```python
from build123d import *

# Parameters (mm, degrees)
EXTRUDE_1_DEPTH     = 115
CUT_EXTRUDE_1_DEPTH = 118.951465627


with BuildPart() as part:
    # 草图1 → 凸台-拉伸1 (new body)
    with BuildSketch(Plane(origin=(0, 0, 0), x_dir=(1, 0, 0), z_dir=(0, 1, 0))):
        with BuildLine():
            Line((-1.042752475, -10.085861632), (3.857247525, -10.085861632))
            ThreePointArc((3.857247525, -10.085861632), (4.757247525, -10.985861632), (3.857247525, -11.885861632))
            Line((3.857247525, -11.885861632), (1.076161722, -11.885861632))
            ThreePointArc((1.076161722, -11.885861632), (0.722608332, -12.032308241), (0.576161722, -12.385861632))
            Line((0.576161722, -12.385861632), (0.576161722, -12.790788968))
            ThreePointArc((0.576161722, -12.790788968), (0.614221956, -12.982130685), (0.722608332, -13.144342359))
            Line((0.722608332, -13.144342359), (2.885447948, -15.307181975))
            ThreePointArc((2.885447948, -15.307181975), (3.858717994, -15.957500229), (5.006768291, -16.185861632))
            Line((5.006768291, -16.185861632), (8.907726758, -16.185861632))
            ThreePointArc((8.907726758, -16.185861632), (10.055777055, -15.957500229), (11.029047102, -15.307181975))
            Line((11.029047102, -15.307181975), (13.191886718, -13.144342359))
            ThreePointArc((13.191886718, -13.144342359), (13.300273094, -12.982130685), (13.338333327, -12.790788968))
            Line((13.338333327, -12.790788968), (13.338333327, -12.385861632))
            ThreePointArc((13.338333327, -12.385861632), (13.191886718, -12.032308241), (12.838333327, -11.885861632))
            Line((12.838333327, -11.885861632), (10.057247525, -11.885861632))
            ThreePointArc((10.057247525, -11.885861632), (9.157247525, -10.985861632), (10.057247525, -10.085861632))
            Line((10.057247525, -10.085861632), (14.957247525, -10.085861632))
            ThreePointArc((14.957247525, -10.085861632), (16.371461087, -10.671648069), (16.957247525, -12.085861632))
            Line((16.957247525, -12.085861632), (16.957247525, -16.985861632))
            ThreePointArc((16.957247525, -16.985861632), (16.057247525, -17.885861632), (15.157247525, -16.985861632))
            Line((15.157247525, -16.985861632), (15.157247525, -14.204775829))
            ThreePointArc((15.157247525, -14.204775829), (15.010800915, -13.851222438), (14.657247525, -13.704775829))
            Line((14.657247525, -13.704775829), (14.252320188, -13.704775829))
            ThreePointArc((14.252320188, -13.704775829), (14.060978472, -13.742836063), (13.898766797, -13.851222438))
            Line((13.898766797, -13.851222438), (11.735927181, -16.014062054))
            ThreePointArc((11.735927181, -16.014062054), (11.085608927, -16.987332101), (10.857247525, -18.135382398))
            Line((10.857247525, -18.135382398), (10.857247525, -22.036340865))
            ThreePointArc((10.857247525, -22.036340865), (11.085608927, -23.184391162), (11.735927181, -24.157661209))
            Line((11.735927181, -24.157661209), (13.898766797, -26.320500825))
            ThreePointArc((13.898766797, -26.320500825), (14.060978472, -26.4288872), (14.252320188, -26.466947434))
            Line((14.252320188, -26.466947434), (14.657247525, -26.466947434))
            ThreePointArc((14.657247525, -26.466947434), (15.010800915, -26.320500825), (15.157247525, -25.966947434))
            Line((15.157247525, -25.966947434), (15.157247525, -23.185861632))
            ThreePointArc((15.157247525, -23.185861632), (16.057247525, -22.285861632), (16.957247525, -23.185861632))
            Line((16.957247525, -23.185861632), (16.957247525, -28.085861632))
            ThreePointArc((16.957247525, -28.085861632), (16.371461087, -29.500075194), (14.957247525, -30.085861632))
            Line((14.957247525, -30.085861632), (10.057247525, -30.085861632))
            ThreePointArc((10.057247525, -30.085861632), (9.157247525, -29.185861632), (10.057247525, -28.285861632))
            Line((10.057247525, -28.285861632), (12.838333327, -28.285861632))
            ThreePointArc((12.838333327, -28.285861632), (13.191886718, -28.139415022), (13.338333327, -27.785861632))
            Line((13.338333327, -27.785861632), (13.338333327, -27.380934295))
            ThreePointArc((13.338333327, -27.380934295), (13.300273094, -27.189592579), (13.191886718, -27.027380904))
            Line((13.191886718, -27.027380904), (11.029047102, -24.864541288))
            ThreePointArc((11.029047102, -24.864541288), (10.055777055, -24.214223034), (8.907726758, -23.985861632))
            Line((8.907726758, -23.985861632), (5.006768291, -23.985861632))
            ThreePointArc((5.006768291, -23.985861632), (3.858717994, -24.214223034), (2.885447948, -24.864541288))
            Line((2.885447948, -24.864541288), (0.722608332, -27.027380904))
            ThreePointArc((0.722608332, -27.027380904), (0.614221956, -27.189592579), (0.576161722, -27.380934295))
            Line((0.576161722, -27.380934295), (0.576161722, -27.785861632))
            ThreePointArc((0.576161722, -27.785861632), (0.722608332, -28.139415022), (1.076161722, -28.285861632))
            Line((1.076161722, -28.285861632), (3.857247525, -28.285861632))
            ThreePointArc((3.857247525, -28.285861632), (4.757247525, -29.185861632), (3.857247525, -30.085861632))
            Line((3.857247525, -30.085861632), (-1.042752475, -30.085861632))
            ThreePointArc((-1.042752475, -30.085861632), (-2.456966038, -29.500075194), (-3.042752475, -28.085861632))
            Line((-3.042752475, -28.085861632), (-3.042752475, -23.185861632))
            ThreePointArc((-3.042752475, -23.185861632), (-2.142752475, -22.285861632), (-1.242752475, -23.185861632))
            Line((-1.242752475, -23.185861632), (-1.242752475, -25.966947434))
            ThreePointArc((-1.242752475, -25.966947434), (-1.096305866, -26.320500825), (-0.742752475, -26.466947434))
            Line((-0.742752475, -26.466947434), (-0.337825138, -26.466947434))
            ThreePointArc((-0.337825138, -26.466947434), (-0.146483422, -26.4288872), (0.015728252, -26.320500825))
            Line((0.015728252, -26.320500825), (2.178567868, -24.157661209))
            ThreePointArc((2.178567868, -24.157661209), (2.828886122, -23.184391162), (3.057247525, -22.036340865))
            Line((3.057247525, -22.036340865), (3.057247525, -18.135382398))
            ThreePointArc((3.057247525, -18.135382398), (2.828886122, -16.987332101), (2.178567868, -16.014062054))
            Line((2.178567868, -16.014062054), (0.015728252, -13.851222438))
            ThreePointArc((0.015728252, -13.851222438), (-0.146483422, -13.742836063), (-0.337825138, -13.704775829))
            Line((-0.337825138, -13.704775829), (-0.742752475, -13.704775829))
            ThreePointArc((-0.742752475, -13.704775829), (-1.096305866, -13.851222438), (-1.242752475, -14.204775829))
            Line((-1.242752475, -14.204775829), (-1.242752475, -16.985861632))
            ThreePointArc((-1.242752475, -16.985861632), (-2.142752475, -17.885861632), (-3.042752475, -16.985861632))
            Line((-3.042752475, -16.985861632), (-3.042752475, -12.085861632))
            ThreePointArc((-3.042752475, -12.085861632), (-2.456966038, -10.671648069), (-1.042752475, -10.085861632))
        make_face()
    extrude(amount=EXTRUDE_1_DEPTH)

    # 草图2 → 切除-拉伸1 (cut, through all)
    with BuildSketch(Plane.XY.offset(30.085861632)):
        Polygon((16.957247525, 115), (-3.042752475, 95), (-3.042752475, 115), align=None)
    extrude(amount=-CUT_EXTRUDE_1_DEPTH, mode=Mode.SUBTRACT)


solid = part.part
```
Source: CAD feature listing. Evaluate the final solid. Frame: model axes, mm. A direction names the side the tool comes from. Give positions to 0.01 mm unless a question says otherwise; leave off trailing zeros.
(1) Material intervals for line 1 along Z through (x, y) = (10, 102); line 2 along Z through (x, y) = (1, 69); line 3 along X through (y, z) = (46.5, 27.25), sorted ascending.
(2) Pull-direction query (Z, two-part tool) for faces 4 (the face through (16.957, 57, 15)), 5 (the face through (11, 55, 11.886)), 6 (the face through (1, 50, 30.086)); classes: +Z half, -Z half, draft (parallel to the pull), parting line (faces both ways), or undercut.
(3) Contact query for flat-ended pins moving along their axis: P1, Ø3, axis at x = 6.5, y = 73, coming from the +Z side; P2, Ø12, axis at x = 10, z = 22, coming from the +Y side; P3, Ø3, axis at x = 4.5, z = 23.5, coming from the -Y side; P4, Ø1.5, axis at y = 83.5, z = 22, coming from the +X side. Output: stop coordinate, or through.
(4) Access query for faces 1 (the face through (3.84, 50.8, 15.95)), 2 (the face through (-3.043, 47, 15)), 3 (the face through (7, 53, 23.986)). Directions: +Z, -Z, +X, -X, +Y, -Y. A direction counts if a zero-diameter tool reaches every point of the face in a straight line with its end or side. Return the directions, or none.
Outcome:
1. line 1: z = 10.09 to 11.88, 15.98 to 24.19, 28.29 to 30.08
1. line 2: z = 10.09 to 11.89, 13.42 to 14.84, 25.34 to 26.75, 28.28 to 30.09
1. line 3: x = -3.04 to 0.59, 13.32 to 16.96
2. face 4: draft
2. face 5: undercut
2. face 6: +Z half
3. P1: stops at z = 23.99
3. P2: stops at y = 114.04
3. P3: stops at y = 0
3. P4: stops at x = 16.84
4. face 1: +Y, -Y
4. face 2: +Z, -Z, -X, +Y, -Y
4. face 3: +Z, +Y, -Y
